Input: part model. Units: mm. Frame: model coordinates. A direction names the side the tool comes from. Round coordinates to 2 decimals unless told otherwise and drop trailing zeros. Loops run counter-clockwise (first coordinate to the right, second up) from the corner with the lowest first, then second, coordinate; pieces in that order, holes last. Notation, with made-up numbers: (24.25, 5) - (41.25, 5) arc R6 cw to (41.25, 9) - close; hole circle Ø7 at (27, 85.25). An arc over 180 degrees is marked (long way). One line per question, with ' | ' between items. Start each with the question number.
Item 1: Section B-B, the plane x = 0. Return loops of the section in (y, z), plus the area to 3 significant figures.
Item 2: Section D-D, the plane z = 5.75. Return loops of the section in (x, y), plus the area to 3 significant figures.
Item 3: Draft query along Y for faces 3 (the face through (-0.1, 26.2, 20)), 4 (the face through (10.17, -17.8, 15.97)), 5 (the face through (-6.94, -31.24, 9.86)). Return one class per face: pulls with the +Y half, pulls with the -Y half, needs draft (parallel to the pull), parting line crosses it, or undercut.
Item 4: Set-up query: faces 1 (the face through (-8, -7, 0)), 2 (the face through (20.5, -0.1, 16)). Return all of +Z, -Z, +X, -X, +Y, -Y with unobstructed straight access to the full face (end or side cutting, diameter ignored); none if empty.
Item 5: Section C-C, the plane y = -9.25. Return loops of the section in (x, z), plus the area to 3 significant figures.
Item 6: Section A-A, the plane y = 0. Return loops of the section in (x, z).
Item 7: Material intervals for line 1 along Y through (x, z) = (0, 16.85); line 2 along Y through (x, z) = (-18.5, 5.5); line 3 along Y through (x, z) = (2, 6.5), sorted ascending.
Item 8: First-contact query: pin 1 (8 mm diameter, centred on y = 25, z = 12, fed in from -X); pin 2 (3 mm diameter, centred on x = -23.5, z = 3.5, fed in from +Y); pin 3 (1 mm diameter, centred on x = 21, z = 4, fed in from -Y); pin 4 (8 mm diameter, centred on x = -3, y = -6.5, fed in from -Z). Flat tips, straight axial feed; report the tip coordinate or a pass-through.
```python
from build123d import *

# Parameters (mm, degrees)
SKETCH1_R           = 32
BOSS_EXTRUDE1_DEPTH = 20
SKETCH2_R           = 26
CUT_EXTRUDE1_DEPTH  = 6
SKETCH3_R           = 20.5
BOSS_EXTRUDE2_DEPTH = 4
SKETCH4_R           = 10
CUT_EXTRUDE2_DEPTH  = 82
SKETCH5_R           = 4.25
CUT_EXTRUDE3_DEPTH  = 19
CIRPATTERN1_COUNT   = 6


with BuildPart() as part:
    # Sketch1 → Boss-Extrude1 (new body)
    with BuildSketch(Plane.XY):
        Circle(SKETCH1_R)
    extrude(amount=BOSS_EXTRUDE1_DEPTH)

    # Sketch2 → Cut-Extrude1 (cut)
    with BuildSketch(Plane.XY.offset(20)):
        Circle(SKETCH2_R)
    extrude(amount=-CUT_EXTRUDE1_DEPTH, mode=Mode.SUBTRACT)

    # Sketch3 → Boss-Extrude2 (add)
    with BuildSketch(Plane.XY.offset(14)):
        Circle(SKETCH3_R)
    extrude(amount=BOSS_EXTRUDE2_DEPTH)

    # Sketch4 → Cut-Extrude2 (cut)
    with BuildSketch(Plane.XY.offset(18)):
        Circle(SKETCH4_R)
    extrude(amount=-CUT_EXTRUDE2_DEPTH, mode=Mode.SUBTRACT)

    # Sketch5 → Cut-Extrude3 (cut, through all)
    with BuildSketch(Plane.XY.offset(18)):
        with Locations((0, 18.5)):
            Circle(SKETCH5_R)
    cut_extrude3 = extrude(amount=-CUT_EXTRUDE3_DEPTH, mode=Mode.SUBTRACT)

    # CirPattern1: Cut-Extrude3 ×6 about axis
    cirpattern1_axis = Axis((0, 0, 0), (0, 0, 1))
    for i in range(1, CIRPATTERN1_COUNT):
        add(cut_extrude3.rotate(cirpattern1_axis, i * 360 / CIRPATTERN1_COUNT), mode=Mode.SUBTRACT)


solid = part.part
```
Return value:
1) outline: (-32, 0) - (-22.75, 0) - (-22.75, 14) - (-26, 14) - (-26, 20) - (-32, 20) - close; (-14.25, 0) - (-10, 0) - (-10, 18) - (-14.25, 18) - close; (10, 0) - (14.25, 0) - (14.25, 18) - (10, 18) - close; (22.75, 0) - (32, 0) - (32, 20) - (26, 20) - (26, 14) - (22.75, 14) - close | area: 484 mm2
2) outline: circle Ø64 at (0, 0); hole circle Ø8.5 at (-16.02, -9.25); hole circle Ø8.5 at (-16.02, 9.25); hole circle Ø20 at (0, 0); hole circle Ø8.5 at (0, -18.5); hole circle Ø8.5 at (0, 18.5); hole circle Ø8.5 at (16.02, -9.25); hole circle Ø8.5 at (16.02, 9.25) | area: 2,560 mm2
3) face 3: needs draft | face 4: undercut | face 5: parting line crosses it
4) face 1: -Z, +X, -X, +Y, -Y | face 2: +Z
5) outline: (-30.63, 0) - (-20.27, 0) - (-20.27, 14) - (-24.3, 14) - (-24.3, 20) - (-30.63, 20) - close; (-11.77, 0) - (-3.8, 0) - (-3.8, 18) - (-11.77, 18) - close; (3.8, 0) - (11.77, 0) - (11.77, 18) - (3.8, 18) - close; (20.27, 0) - (30.63, 0) - (30.63, 20) - (24.3, 20) - (24.3, 14) - (20.27, 14) - close | area: 653 mm2
6) outline: (-32, 0) - (-10, 0) - (-10, 18) - (-20.5, 18) - (-20.5, 14) - (-26, 14) - (-26, 20) - (-32, 20) - close; (10, 0) - (32, 0) - (32, 20) - (26, 20) - (26, 14) - (20.5, 14) - (20.5, 18) - (10, 18) - close
7) line 1: -32 to -26, -14.25 to -10, 10 to 14.25, 26 to 32 | line 2: -26.11 to -12.7, -5.8 to 5.8, 12.7 to 26.11 | line 3: -31.94 to -22.25, -14.75 to -9.8, 9.8 to 14.75, 22.25 to 31.94
8) pin 1: x = -24.15 | pin 2: y = 23.24 | pin 3: y = -24.57 | pin 4: z = 0
